CAD build for the part. Positions are in the model's coordinates, mm. A direction names the side the tool comes from. Give positions to 0.01 mm unless a question says otherwise; leave off trailing zeros. Loops run counter-clockwise (first coordinate to the right, second up) from the corner with the lowest first, then second, coordinate; pieces in that order, holes last. Notation, with made-up numbers: (4, 1.25) - (56, 1.25) arc R7 ccw to (56, 14.25) - close; hole circle Ø3 at (-39.5, 38.25). An arc over 180 degrees is marked (long way). Return JSON: item names as keys, results as strings.
from build123d import *

# Parameters (mm, degrees)
SKETCH1_R           = 3.36
BOSS_EXTRUDE1_DEPTH = 1.86
BOSS_EXTRUDE1_TAPER = 20
SKETCH2_R           = 1.5
BOSS_EXTRUDE2_DEPTH = 18.14
CUT_EXTRUDE1_DEPTH  = 1.5


with BuildPart() as part:
    # Sketch1 → Boss-Extrude1 (new body)
    with BuildSketch(Plane(origin=(0, 0, 0), x_dir=(1, 0, 0), z_dir=(0, 1, 0))):
        Circle(SKETCH1_R)
    extrude(amount=BOSS_EXTRUDE1_DEPTH, taper=BOSS_EXTRUDE1_TAPER)

    # Sketch2 → Boss-Extrude2 (add)
    with BuildSketch(Plane(origin=(0, 1.86, 0), x_dir=(1, 0, 0), z_dir=(0, 1, 0))):
        with Locations(Location((0, 0, 0), (0, 0, 270))):
            Circle(SKETCH2_R)
    extrude(amount=BOSS_EXTRUDE2_DEPTH)

    # Sketch3 → Cut-Extrude1 (cut)
    with BuildSketch(Plane.XZ):
        Polygon((0, 1.154700538), (-1, 0.577350269), (-1, -0.577350269), (0, -1.154700538), (1, -0.577350269), (1, 0.577350269), align=None)
    extrude(amount=-CUT_EXTRUDE1_DEPTH, mode=Mode.SUBTRACT)


solid = part.part
1. Which spindle directions (+Z, -Z, +X, -X, +Y, -Y) get a long thin tool onto all of the face, cutting with end or side? Do faces 5 (the face through (0, 20, 0)), 6 (the face through (-0.49, 0.74, 0.87)). Say none if no direction does.
Values follow:
{"face 5": "+Z, -Z, +X, -X, +Y", "face 6": "-Y"}
2. Drop flat-ended pins along their axis: P1, Ø1, axis at x = -0.5, y = 13, coming from the +Z side; P2, Ø1.5, axis at x = -2, y = 14, coming from the -Z side; P3, Ø0.9, axis at y = 0.5, z = 0, coming from the -X side. Give the stop position or say it passes through.
Values follow:
{"P1": "stops at z = 1.5", "P2": "stops at z = -0.83", "P3": "stops at x = -3.34"}
3. Drill centre lines: probe 1 along Y at (x, z) = (-0.5, -1.75); probe 2 along Y at (x, z) = (0.25, 0); probe 3 along Z at (x, y) = (0.5, 1). Where is each one in solid material? Low to high.
Values follow:
{"probe 1": "y = 0 to 1.86", "probe 2": "y = 1.5 to 20", "probe 3": "z = -2.95 to -0.87, 0.87 to 2.95"}
4. Pull direction Z, two halves, no side cores. Call faces 1 (the face through (0.51, 0.74, 0.86)), 2 (the face through (0.45, 10.8, 1.43)), 3 (the face through (1.2, 1.86, 1.2)), 4 (the face through (-0.51, 0.74, -0.86)): +Z half, -Z half, draft (parallel to the pull), parting line (faces both ways), or undercut.
Values follow:
{"face 1": "undercut", "face 2": "parting line", "face 3": "draft", "face 4": "undercut"}
5. Cut at A-A, the plane y = 12.25. Write the cut outline in (x, z).
Values follow:
{"outline": "circle Ø3 at (0, 0)"}
